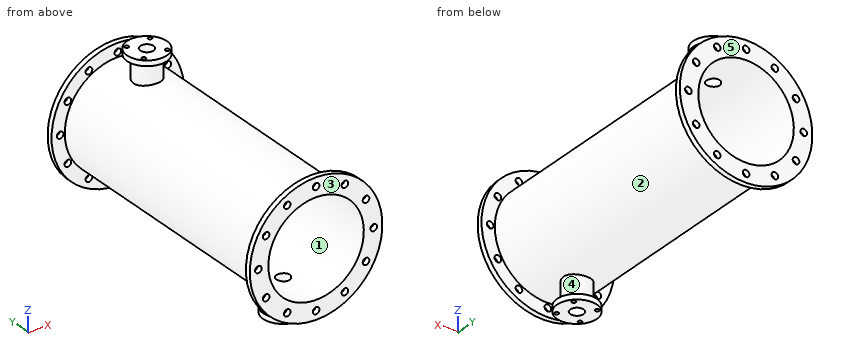
from build123d import *

# Parameters (mm, degrees)
SKETCH1_R                = 250
SKETCH1_R_2              = 12.5
BOSS_EXTRUDE1_DEPTH      = 20
SKETCH2_R                = 200
BOSS_EXTRUDE2_DEPTH      = 1000
SKETCH3_R                = 250
SKETCH3_R_2              = 12.5
BOSS_EXTRUDE3_DEPTH      = 20
SKETCH4_R                = 180
CUT_EXTRUDE1_DEPTH       = 1040
BOSS_EXTRUDE5_DEPTH      = 80
BOSS_EXTRUDE5_DEPTH_BACK = 10
SKETCH6_R                = 50
SKETCH7_R                = 75
SKETCH7_R_2              = 7.5
BOSS_EXTRUDE6_DEPTH      = 20
SKETCH8_R                = 25
CUT_EXTRUDE2_DEPTH       = 142
BOSS_EXTRUDE7_DEPTH      = 80
BOSS_EXTRUDE7_DEPTH_BACK = 13
SKETCH9_R                = 50
SKETCH10_R               = 75
SKETCH10_R_2             = 7.5
BOSS_EXTRUDE8_DEPTH      = 20
SKETCH11_R               = 25
CUT_EXTRUDE3_DEPTH       = 145


with BuildPart() as part:
    # Sketch1 → Boss-Extrude1 (new body)
    with BuildSketch(Plane(origin=(0, 0, 0), x_dir=(1, 0, 0), z_dir=(0, 1, 0))):
        with Locations(Location((0, 0, 0), (0, 0, 270))):
            Circle(SKETCH1_R)
        with Locations(Location((0, 217.5, 0), (0, 0, 270))):
            Circle(SKETCH1_R_2, mode=Mode.SUBTRACT)
        with Locations(Location((108.75, 188.360525323, 0), (0, 0, 270))):
            Circle(SKETCH1_R_2, mode=Mode.SUBTRACT)
        with Locations(Location((188.360525323, 108.75, 0), (0, 0, 270))):
            Circle(SKETCH1_R_2, mode=Mode.SUBTRACT)
        with Locations(Location((217.5, 0, 0), (0, 0, 270))):
            Circle(SKETCH1_R_2, mode=Mode.SUBTRACT)
        with Locations(Location((188.360525323, -108.75, 0), (0, 0, 270))):
            Circle(SKETCH1_R_2, mode=Mode.SUBTRACT)
        with Locations(Location((108.75, -188.360525323, 0), (0, 0, 270))):
            Circle(SKETCH1_R_2, mode=Mode.SUBTRACT)
        with Locations(Location((0, -217.5, 0), (0, 0, 270))):
            Circle(SKETCH1_R_2, mode=Mode.SUBTRACT)
        with Locations(Location((-108.75, -188.360525323, 0), (0, 0, 270))):
            Circle(SKETCH1_R_2, mode=Mode.SUBTRACT)
        with Locations(Location((-188.360525323, -108.75, 0), (0, 0, 270))):
            Circle(SKETCH1_R_2, mode=Mode.SUBTRACT)
        with Locations(Location((-217.5, 0, 0), (0, 0, 270))):
            Circle(SKETCH1_R_2, mode=Mode.SUBTRACT)
        with Locations(Location((-188.360525323, 108.75, 0), (0, 0, 270))):
            Circle(SKETCH1_R_2, mode=Mode.SUBTRACT)
        with Locations(Location((-108.75, 188.360525323, 0), (0, 0, 270))):
            Circle(SKETCH1_R_2, mode=Mode.SUBTRACT)
    extrude(amount=BOSS_EXTRUDE1_DEPTH)

    # Sketch2 → Boss-Extrude2 (add)
    with BuildSketch(Plane(origin=(0, 20, 0), x_dir=(1, 0, 0), z_dir=(0, 1, 0))):
        with Locations(Location((0, 0, 0), (0, 0, 270))):
            Circle(SKETCH2_R)
    extrude(amount=BOSS_EXTRUDE2_DEPTH)

    # Sketch3 → Boss-Extrude3 (add)
    with BuildSketch(Plane(origin=(0, 1020, 0), x_dir=(1, 0, 0), z_dir=(0, 1, 0))):
        with Locations(Location((0, 0, 0), (0, 0, 270))):
            Circle(SKETCH3_R)
        with Locations(Location((0, 217.5, 0), (0, 0, 270))):
            Circle(SKETCH3_R_2, mode=Mode.SUBTRACT)
        with Locations(Location((108.75, 188.360525323, 0), (0, 0, 270))):
            Circle(SKETCH3_R_2, mode=Mode.SUBTRACT)
        with Locations(Location((188.360525323, 108.75, 0), (0, 0, 270))):
            Circle(SKETCH3_R_2, mode=Mode.SUBTRACT)
        with Locations(Location((217.5, 0, 0), (0, 0, 270))):
            Circle(SKETCH3_R_2, mode=Mode.SUBTRACT)
        with Locations(Location((188.360525323, -108.75, 0), (0, 0, 270))):
            Circle(SKETCH3_R_2, mode=Mode.SUBTRACT)
        with Locations(Location((108.75, -188.360525323, 0), (0, 0, 270))):
            Circle(SKETCH3_R_2, mode=Mode.SUBTRACT)
        with Locations(Location((0, -217.5, 0), (0, 0, 270))):
            Circle(SKETCH3_R_2, mode=Mode.SUBTRACT)
        with Locations(Location((-108.75, -188.360525323, 0), (0, 0, 270))):
            Circle(SKETCH3_R_2, mode=Mode.SUBTRACT)
        with Locations(Location((-188.360525323, -108.75, 0), (0, 0, 270))):
            Circle(SKETCH3_R_2, mode=Mode.SUBTRACT)
        with Locations(Location((-217.5, 0, 0), (0, 0, 270))):
            Circle(SKETCH3_R_2, mode=Mode.SUBTRACT)
        with Locations(Location((-188.360525323, 108.75, 0), (0, 0, 270))):
            Circle(SKETCH3_R_2, mode=Mode.SUBTRACT)
        with Locations(Location((-108.75, 188.360525323, 0), (0, 0, 270))):
            Circle(SKETCH3_R_2, mode=Mode.SUBTRACT)
    extrude(amount=BOSS_EXTRUDE3_DEPTH)

    # Sketch4 → Cut-Extrude1 (cut)
    with BuildSketch(Plane(origin=(0, 1040, 0), x_dir=(1, 0, 0), z_dir=(0, 1, 0))):
        with Locations(Location((0, 0, 0), (0, 0, 270))):
            Circle(SKETCH4_R)
    extrude(amount=-CUT_EXTRUDE1_DEPTH, mode=Mode.SUBTRACT)

    # Sketch6 → Boss-Extrude5 (add, two sides: drawn at the far end of the back side and taken through both)
    with BuildSketch(Plane(origin=(0, 0, -200), x_dir=(-1, 0, 0), z_dir=(0, 0, -1)).offset(-BOSS_EXTRUDE5_DEPTH_BACK)):
        with Locations((0, 170)):
            Circle(SKETCH6_R)
    extrude(amount=BOSS_EXTRUDE5_DEPTH + BOSS_EXTRUDE5_DEPTH_BACK)

    # Sketch7 → Boss-Extrude6 (add)
    with BuildSketch(Plane(origin=(0, 0, -280), x_dir=(-1, 0, 0), z_dir=(0, 0, -1))):
        with Locations((0, 170)):
            Circle(SKETCH7_R)
        with Locations((44.194173824, 214.194173824)):
            Circle(SKETCH7_R_2, mode=Mode.SUBTRACT)
        with Locations((44.194173824, 125.805826176)):
            Circle(SKETCH7_R_2, mode=Mode.SUBTRACT)
        with Locations((-44.194173824, 125.805826176)):
            Circle(SKETCH7_R_2, mode=Mode.SUBTRACT)
        with Locations((-44.194173824, 214.194173824)):
            Circle(SKETCH7_R_2, mode=Mode.SUBTRACT)
    extrude(amount=BOSS_EXTRUDE6_DEPTH)

    # Sketch8 → Cut-Extrude2 (cut)
    with BuildSketch(Plane(origin=(0, 0, -300), x_dir=(-1, 0, 0), z_dir=(0, 0, -1))):
        with Locations((0, 170)):
            Circle(SKETCH8_R)
    extrude(amount=-CUT_EXTRUDE2_DEPTH, mode=Mode.SUBTRACT)

    # Sketch9 → Boss-Extrude7 (add, two sides: drawn at the far end of the back side and taken through both)
    with BuildSketch(Plane.XY.offset(200).offset(-BOSS_EXTRUDE7_DEPTH_BACK)):
        with Locations((0, 870)):
            Circle(SKETCH9_R)
    extrude(amount=BOSS_EXTRUDE7_DEPTH + BOSS_EXTRUDE7_DEPTH_BACK)

    # Sketch10 → Boss-Extrude8 (add)
    with BuildSketch(Plane.XY.offset(280)):
        with Locations((0, 870)):
            Circle(SKETCH10_R)
        with Locations((44.194173824, 914.194173824)):
            Circle(SKETCH10_R_2, mode=Mode.SUBTRACT)
        with Locations((44.194173824, 825.805826176)):
            Circle(SKETCH10_R_2, mode=Mode.SUBTRACT)
        with Locations((-44.194173824, 825.805826176)):
            Circle(SKETCH10_R_2, mode=Mode.SUBTRACT)
        with Locations((-44.194173824, 914.194173824)):
            Circle(SKETCH10_R_2, mode=Mode.SUBTRACT)
    extrude(amount=BOSS_EXTRUDE8_DEPTH)

    # Sketch11 → Cut-Extrude3 (cut)
    with BuildSketch(Plane.XY.offset(300)):
        with Locations((0, 870)):
            Circle(SKETCH11_R)
    extrude(amount=-CUT_EXTRUDE3_DEPTH, mode=Mode.SUBTRACT)


solid = part.part
The listing builds one solid part. Answer for the finished solid, in the listing's coordinates (mm). Face numbers are marked on the shaded views. A direction names the side the tool comes from. Give positions to 0.01 mm unless a question says otherwise; leave off trailing zeros. Write each loop counter-clockwise with the first axis right and the second up, starting at its lowest first coordinate (ties: lowest second). Pieces come first, ordered by that corner, then holes. Notation, with made-up numbers: (81.5, 65.25) - (114.5, 65.25) arc R20 cw to (114.5, 75.25) - close; hole circle Ø8 at (-32.75, 0.5). An arc over 180 degrees is marked (long way). Use a Markdown table: item, result.
1. For a pull along Y with two mould halves and no side action, classify the marked faces 3, 4 and 5 as released by +Y, released by -Y, zero draft, split by the parting line, or undercut.
Values follow:
| item | result |
|---|---|
| face 3 | released by -Y |
| face 4 | undercut |
| face 5 | released by +Y |
2. A tool of negligible diameter and unlimited length cuts with its end or side. For the marked faces 1 and 2, from which of +Z, -Z, +X, -X, +Y, -Y can it reach the whole face along a straight path? Write none if from no direction.
Values follow:
| item | result |
|---|---|
| face 1 | +Y, -Y |
| face 2 | none |
3. Section B-B on x = -217.5 is taken. Write down the section's boundary in (y, z), plus the area to 3 significant figures.
Values follow:
| item | result |
|---|---|
| outline | (0, -123.26) - (20, -123.26) - (20, -12.5) - (0, -12.5) - close; (0, 12.5) - (20, 12.5) - (20, 123.26) - (0, 123.26) - close; (1020, -123.26) - (1040, -123.26) - (1040, -12.5) - (1020, -12.5) - close; (1020, 12.5) - (1040, 12.5) - (1040, 123.26) - (1020, 123.26) - close |
| area | 8,860 mm² |
4. Find the intervals of material crossed by probe 1 along Y at (x, z) = (-114, -218.5); probe 2 along Y at (x, z) = (-18.5, 220); probe 3 along X at (y, z) = (1024, -108), in increasing order. Write a range as from..to.
Values follow:
| item | result |
|---|---|
| probe 1 | y = 0..20, 1020..1040 |
| probe 2 | y = 0..20, 823.55..853.18, 886.82..916.45, 1020..1040 |
| probe 3 | x = -225.47..-200.84, -175.88..-144, 144..175.88, 200.84..225.47 |
5. Section A-A on z = 217.5 is taken. Write down the section's boundary in (x, y), plus the area to 3 significant figures.
Values follow:
| item | result |
|---|---|
| outline | (-123.26, 0) - (-12.5, 0) - (-12.5, 20) - (-123.26, 20) - close; (-123.26, 1020) - (-12.5, 1020) - (-12.5, 1040) - (-123.26, 1040) - close; circle Ø100 at (0, 870); (12.5, 0) - (123.26, 0) - (123.26, 20) - (12.5, 20) - close; (12.5, 1020) - (123.26, 1020) - (123.26, 1040) - (12.5, 1040) - close; hole circle Ø50 at (0, 870) |
| area | 14,800 mm² |
6. Section C-C on z = 0 is taken. Count the separate pieces of the cut face and the enclosed holes in it, plus the area to 3 significant figures.
Values follow:
| item | result |
|---|---|
| separate pieces | 6 |
| enclosed holes | 0 |
| area | 43,600 mm² |
7. Section D-D on y = 306 is taken. Write down the section's boundary in (x, z).
Values follow:
| item | result |
|---|---|
| outline | circle Ø400 at (0, 0); hole circle Ø360 at (0, 0) |
8. Each of these flat-tipped pins is pushed along its axis until it touches: P1, Ø5, axis at x = -50, y = 665.5, coming from the -Z side; P2, Ø5, axis at x = 105, y = 702, coming from the +Z side; P3, Ø2, axis at x = 145, y = 467, coming from the -Z side. Where does it stop, or does it pass through?
Values follow:
| item | result |
|---|---|
| P1 | stops at z = -194.28 |
| P2 | stops at z = 171.74 |
| P3 | stops at z = -138.79 |
